The model under review builds one solid part; all positions refer to its coordinate system, in mm. Face numbers are marked on the shaded views. A direction names the side the tool comes from. Coordinates: 2 decimals unless noted, no trailing zeros. Loops run counter-clockwise (first coordinate to the right, second up) from the corner with the lowest first, then second, coordinate; pieces in that order, holes last. Notation, with made-up numbers: M -30.5,-36 L -5.5,-36 A31 cw -5.5,-8 Z; hole C 82.5,26 d2. An arc over 180 degrees is marked long. Write item = value, one per line. Start each with the question number.
Q1. Clearance check with a flat-ended pin moving along its axis: pin 1 Ø2 at (y, z) = (-1.5, 9.5) entering from +X. State where the tip first meets the part, or that it passes through.
Q2. We need section A-A on x = 0. Give the boundary of the cut face in (y, z), and give its area (3 significant figures).
Q3. Wall thickness on probe 1 along Z at (x, y) = (-1.85, -0.1); probe 2 along X at (y, z) = (0.1, 14.75); probe 3 along X at (y, z) = (1.2, 22.25): over which ranges is each line inside the solid? List them lowest first.
Q4. We need section C-C on z = 20.5. Give the boundary of the cut face in (x, y), and give its area (3 significant figures).
Q5. For the marked faces 1 and 2, list the 3-axis set-ups (+Z, -Z, +X, -X, +Y, -Y) from which the entire face can be reached by the end or side of a thin tool; tool diameter is ignored.
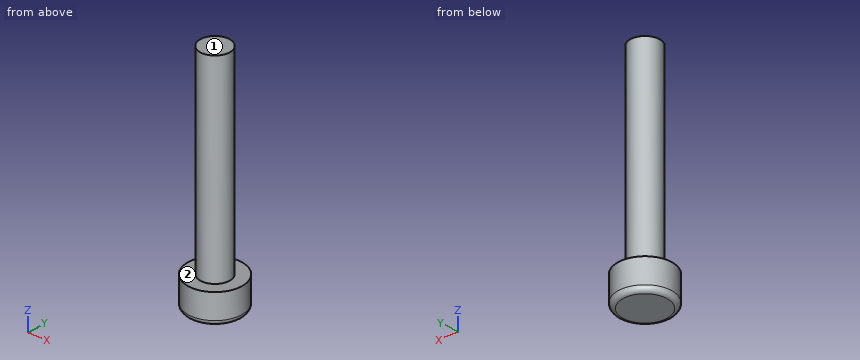
from build123d import *

# Parameters (mm, degrees)
SKETCH_2_R      = 2.75
EXTRUDE_1_DEPTH = 3
SKETCH_3_R      = 1.5
EXTRUDE_2_DEPTH = 20
FILLET_1_R      = 0.5


with BuildPart() as part:
    # ｽｹｯﾁ2 → ﾎﾞｽ - 押し出し1 (new body)
    with BuildSketch(Plane.XY):
        Circle(SKETCH_2_R)
    extrude(amount=EXTRUDE_1_DEPTH)

    # ｽｹｯﾁ3 → ﾎﾞｽ - 押し出し2 (add)
    with BuildSketch(Plane.XY.offset(3)):
        Circle(SKETCH_3_R)
    extrude(amount=EXTRUDE_2_DEPTH)

    # ﾌｨﾚｯﾄ1
    fillet_1_edges = [part.edges().sort_by_distance(p)[0] for p in [
        (-2.75, 0, 0),
    ]]
    fillet(fillet_1_edges, radius=FILLET_1_R)


solid = part.part
Returned:
q1.pin_1 = 1.41
q2.outline = M -2.75,0.5 A0.5 ccw -2.25,0 L 2.25,0 A0.5 ccw 2.75,0.5 L 2.75,3 L 1.5,3 L 1.5,23 L -1.5,23 L -1.5,3 L -2.75,3 Z
q2.area = 76.4 mm^2
q3.probe_1 = 0 to 3
q3.probe_2 = -1.5 to 1.5
q3.probe_3 = -0.9 to 0.9
q4.outline = C 0,0 d3
q4.area = 7.07 mm^2
q5.face_1 = +Z, +X, -X, +Y, -Y
q5.face_2 = +Z
